Geometry check sheet. Reference: the model listing, model coordinates, mm. A direction names the side the tool comes from. Give positions to 0.01 mm unless a question says otherwise; leave off trailing zeros. Order: outer loops, then holes, each group sorted by start corner. A loop starts at its lowest first (then second) coordinate and runs counter-clockwise, first axis right, second up. Notation, with made-up numbers: M 52,13 L 76,13 A13 ccw 76,18 Z; hole C 41.5,21.5 d1. An arc over 180 degrees is marked long. Answer as CSV lines item,"result". Start each with the question number.
```python
from build123d import *

# Parameters (mm, degrees)
ESBO_O1_W                 = 72.5
ESBO_O1_H                 = 39.5
RESSALTO_EXTRUS_O1_DEPTH  = 2
ESBO_O1_3_W               = 78.5
ESBO_O1_3_H               = 45.5
ESBO_O1_3_W_2             = 72.5
ESBO_O1_3_H_2             = 39.5
RESSALTO_EXTRUS_O2_DEPTH  = 12
ESBO_O1_4_W               = 10.25
ESBO_O1_4_H               = 12
ESBO_O1_4_R               = 1.6
RESSALTO_EXTRUS_O3_DEPTH  = 6
ESBO_O3_W                 = 9.7
ESBO_O3_H                 = 3.2
RESSALTO_EXTRUS_O4_DEPTH  = 3.5
ESBO_O5_W                 = 3.952514159
ESBO_O5_H                 = 45.5
CORTE_EXTRUS_O4_DEPTH     = 3
RESSALTO_EXTRUS_O5_DEPTH  = 9.7
RESSALTO_EXTRUS_O6_DEPTH  = 9.7
ESBO_O9_W                 = 79.78598512
ESBO_O9_H                 = 21.194293461
CORTE_EXTRUS_O5_DEPTH     = 10
ESBO_O11_W                = 10.25
ESBO_O11_H                = 12
RESSALTO_EXTRUS_O8_DEPTH  = 1.2
ESBO_O12_R                = 1.6
CORTE_EXTRUS_O6_DEPTH     = 99.200369144
CORTE_EXTRUS_O7_START     = -3.75
ESBO_O13_R                = 1.6
CORTE_EXTRUS_O7_DEPTH     = 3.75
ESBO_O14_W                = 10.25
ESBO_O14_H                = 12
RESSALTO_EXTRUS_O10_DEPTH = 2


with BuildPart() as part:
    # Esboço1 → Ressalto-extrusão1 (new body)
    with BuildSketch(Plane.XY):
        with Locations((-36.25, 19.75)):
            Rectangle(ESBO_O1_W, ESBO_O1_H)
    extrude(amount=RESSALTO_EXTRUS_O1_DEPTH)

    # Esboço1<3> → Ressalto-extrusão2 (add)
    with BuildSketch(Plane.XY):
        with Locations((-36.25, 19.75)):
            Rectangle(ESBO_O1_3_W, ESBO_O1_3_H)
        with Locations((-36.25, 19.75)):
            Rectangle(ESBO_O1_3_W_2, ESBO_O1_3_H_2, mode=Mode.SUBTRACT)
    extrude(amount=RESSALTO_EXTRUS_O2_DEPTH)

    # Esboço1<4> → Ressalto-extrusão3 (add)
    # profile 1 of 2: a face of its own
    with BuildSketch(Plane.XY):
        with Locations((-80.625, 10.5)):
            Rectangle(ESBO_O1_4_W, ESBO_O1_4_H)
        with Locations((-79.75, 10.5)):
            Circle(ESBO_O1_4_R, mode=Mode.SUBTRACT)
    # profile 2 of 2: a face of its own
    with BuildSketch(Plane.XY):
        with Locations((8.125, 10.5)):
            Rectangle(ESBO_O1_4_W, ESBO_O1_4_H)
        with Locations((7.25, 10.5)):
            Circle(ESBO_O1_4_R, mode=Mode.SUBTRACT)
    extrude(amount=RESSALTO_EXTRUS_O3_DEPTH)

    # Esboço3 → Ressalto-extrusão4 (add)
    with BuildSketch(Plane(origin=(0, 0, 0), x_dir=(-1, 0, 0), z_dir=(0, 0, -1))):
        with Locations((63.4, 24.1)):
            Rectangle(ESBO_O3_W, ESBO_O3_H)
        with Locations((9.1, 24.1)):
            Rectangle(ESBO_O3_W, ESBO_O3_H)
    extrude(amount=RESSALTO_EXTRUS_O4_DEPTH)

    # Esboço5 → Corte-extrusão4 (cut)
    with BuildSketch(Plane(origin=(0, 0, 0), x_dir=(-1, 0, 0), z_dir=(0, 0, -1))):
        with Locations((36.22625708, 19.75)):
            Rectangle(ESBO_O5_W, ESBO_O5_H)
    extrude(amount=-CORTE_EXTRUS_O4_DEPTH, mode=Mode.SUBTRACT)

    # Esboço7 → Ressalto-extrusão5 (add)
    with BuildSketch(Plane(origin=(-58.55, 0, 0), x_dir=(0, 0, -1), z_dir=(1, 0, 0))):
        Polygon((3.5, 25.7), (3.5, 26.2), (4.5, 25.7), (3.5, 22.5), align=None)
    extrude(amount=-RESSALTO_EXTRUS_O5_DEPTH)

    # Esboço8 → Ressalto-extrusão6 (add)
    with BuildSketch(Plane(origin=(-4.25, 0, 0), x_dir=(0, 0, -1), z_dir=(1, 0, 0))):
        Polygon((3.5, 25.7), (3.5, 26.2), (4.5, 25.7), (3.5, 22.5), align=None)
    extrude(amount=-RESSALTO_EXTRUS_O6_DEPTH)

    # Esboço9 → Corte-extrusão5 (cut)
    with BuildSketch(Plane(origin=(0, 0, -10), x_dir=(-1, 0, 0), z_dir=(0, 0, -1))):
        with Locations((37.346022271, 20.867499613)):
            Rectangle(ESBO_O9_W, ESBO_O9_H)
    extrude(amount=-CORTE_EXTRUS_O5_DEPTH, mode=Mode.SUBTRACT)

    # Esboço11 → Ressalto-extrusão8 (add)
    with BuildSketch(Plane.XY.offset(6)):
        with Locations((8.125, 10.5)):
            Rectangle(ESBO_O11_W, ESBO_O11_H)
        with Locations((-80.625, 10.5)):
            Rectangle(ESBO_O11_W, ESBO_O11_H)
    extrude(amount=RESSALTO_EXTRUS_O8_DEPTH)

    # Esboço12 → Corte-extrusão6 (cut, through all)
    with BuildSketch(Plane(origin=(0, 0, -10), x_dir=(-1, 0, 0), z_dir=(0, 0, -1))):
        with Locations(Location((-7.25, 10.5, 0), (0, 0, 180))):
            Circle(ESBO_O12_R)
        with Locations(Location((79.75, 10.5, 0), (0, 0, 180))):
            Circle(ESBO_O12_R)
    extrude(amount=-CORTE_EXTRUS_O6_DEPTH, mode=Mode.SUBTRACT)

    # Esboço13 → Corte-extrusão7 (cut)
    # profile 1 of 2: a face of its own
    with BuildSketch(Plane.XY.offset(7.2).offset(CORTE_EXTRUS_O7_START)):
        Polygon((-83.214101615, 10.5), (-81.482050808, 7.5), (-78.017949192, 7.5), (-76.285898385, 10.5), (-78.017949192, 13.5), (-81.482050808, 13.5), align=None)
        with Locations((-79.75, 10.5)):
            Circle(ESBO_O13_R, mode=Mode.SUBTRACT)
    # profile 2 of 2: a face of its own
    with BuildSketch(Plane.XY.offset(7.2).offset(CORTE_EXTRUS_O7_START)):
        Polygon((10.714101615, 10.5), (8.982050808, 13.5), (5.517949192, 13.5), (3.785898385, 10.5), (5.517949192, 7.5), (8.982050808, 7.5), align=None)
        with Locations((7.25, 10.5)):
            Circle(ESBO_O13_R, mode=Mode.SUBTRACT)
    extrude(amount=CORTE_EXTRUS_O7_DEPTH, mode=Mode.SUBTRACT)

    # Esboço14 → Ressalto-extrusão10 (add)
    # profile 1 of 2: a face of its own
    with BuildSketch(Plane.XY.offset(7.2)):
        with Locations((8.125, 10.5)):
            Rectangle(ESBO_O14_W, ESBO_O14_H)
        Polygon((8.982050808, 7.5), (10.714101615, 10.5), (8.982050808, 13.5), (5.517949192, 13.5), (3.785898385, 10.5), (5.517949192, 7.5), align=None, mode=Mode.SUBTRACT)
    # profile 2 of 2: a face of its own
    with BuildSketch(Plane.XY.offset(7.2)):
        with Locations((-80.625, 10.5)):
            Rectangle(ESBO_O14_W, ESBO_O14_H)
        Polygon((-81.482050808, 13.5), (-83.214101615, 10.5), (-81.482050808, 7.5), (-78.017949192, 7.5), (-76.285898385, 10.5), (-78.017949192, 13.5), align=None, mode=Mode.SUBTRACT)
    extrude(amount=RESSALTO_EXTRUS_O10_DEPTH)


solid = part.part
```
Item 1: Section check B-B on x = 7.25. Record the boundary of the cut face in (y, z), then the cut area to 3 significant figures.
Item 2: Draft check along X on faces 1 (the face through (-77.164, 8.979, 6.285)), 2 (the face through (8, 4.5, 5)), 3 (the face through (13.25, 10, 5)), 4 (the face through (-85.75, 10, 5)). Enter one of: pulls with the +X half, pulls with the -X half, needs draft (parallel to the pull), parting line crosses it, or undercut.
Item 3: Section check C-C on z = 7.75. Record the boundary of the cut face in (x, y).
Item 4: Access from +Z, -Z, +X, -X, +Y, -Y to the whole of each face (thin tool, end or side, straight path). Record for faces 5 (the face through (-39.3, -0.4, 12)), 6 (the face through (-36, -1, 3)), 7 (the face through (10.3, 11.9, 9.2)), 8 (the face through (-37, 39.5, 7)).
Item 5: Section check D-D on x = -8. Record the boundary of the cut face in (y, z).
Item 6: Section check A-A on y = 19. Record the boundary of the cut face in (x, z).
Item 7: Scan lines: line 1 along X through (y, z) = (22.5, 6); line 2 along Y through (x, z) = (-39, 8.25); line 3 along Y through (x, z) = (7.25, 2.3). Record each from-to range of solid material in increasing order.
Item 8: Depth check by flat-ended pin: pin 1 Ø3.5 at (y, z) = (22.5, 1) entering from +X; pin 2 Ø1 at (x, z) = (-80.5, 7.5) entering from +Y; pin 3 Ø0.9 at (y, z) = (20.5, 1.5) entering from -X; pin 4 Ø1.8 at (x, y) = (7.5, 10.5) entering from +Z. Enter the tip coordinate at first touch or a pass-through.
Numbers:
1,outline,"M 4.5,0 L 8.9,0 L 8.9,3.45 L 7.5,3.45 L 7.5,9.2 L 4.5,9.2 Z; M 12.1,0 L 16.5,0 L 16.5,9.2 L 13.5,9.2 L 13.5,3.45 L 12.1,3.45 Z"
1,area,"64.9 mm2"
2,face 1,"undercut"
2,face 2,"needs draft"
2,face 3,"pulls with the +X half"
2,face 4,"pulls with the -X half"
3,outline,"M -85.75,4.5 L -75.5,4.5 L -75.5,-3 L 3,-3 L 3,4.5 L 13.25,4.5 L 13.25,16.5 L 3,16.5 L 3,42.5 L -75.5,42.5 L -75.5,16.5 L -85.75,16.5 Z; hole M -83.21,10.5 L -81.48,7.5 L -78.02,7.5 L -76.29,10.5 L -78.02,13.5 L -81.48,13.5 Z; hole M -72.5,0 L 0,0 L 0,39.5 L -72.5,39.5 Z; hole M 3.79,10.5 L 5.52,7.5 L 8.98,7.5 L 10.71,10.5 L 8.98,13.5 L 5.52,13.5 Z"
4,face 5,"+Z, +X, -X, +Y, -Y"
4,face 6,"-Z, +Y, -Y"
4,face 7,"+Z, +X, +Y, -Y"
4,face 8,"+Z"
5,outline,"M -3,0 L 42.5,0 L 42.5,12 L 39.5,12 L 39.5,2 L 0,2 L 0,12 L -3,12 Z"
6,outline,"M -75.5,0 L -38.2,0 L -38.2,2 L -72.5,2 L -72.5,12 L -75.5,12 Z; M -34.25,0 L 3,0 L 3,12 L 0,12 L 0,2 L -34.25,2 Z"
7,line 1,"-75.5 to -72.5, 0 to 3"
7,line 2,"-3 to 0, 39.5 to 42.5"
7,line 3,"4.5 to 8.9, 12.1 to 16.5"
8,pin 1,"x = 3"
8,pin 2,"y = 16.5"
8,pin 3,"x = -75.5"
8,pin 4,"through"
